Here's the drawing with two shaded views (mm, measured from the low corner). I have some questions. Coordinates: 2 decimals unless noted, no trailing zeros. Loops run counter-clockwise (first coordinate to the right, second up) from the corner with the lowest first, then second, coordinate; pieces in that order, holes last. Notation, with made-up numbers: M 42.5,43.5 L 80.5,43.5 A20 cw 80.5,50.5 Z; hole C 88.25,-2 d6. An arc over 180 degrees is marked long. Return JSON: item names as keys, results as strings. Group by question number.
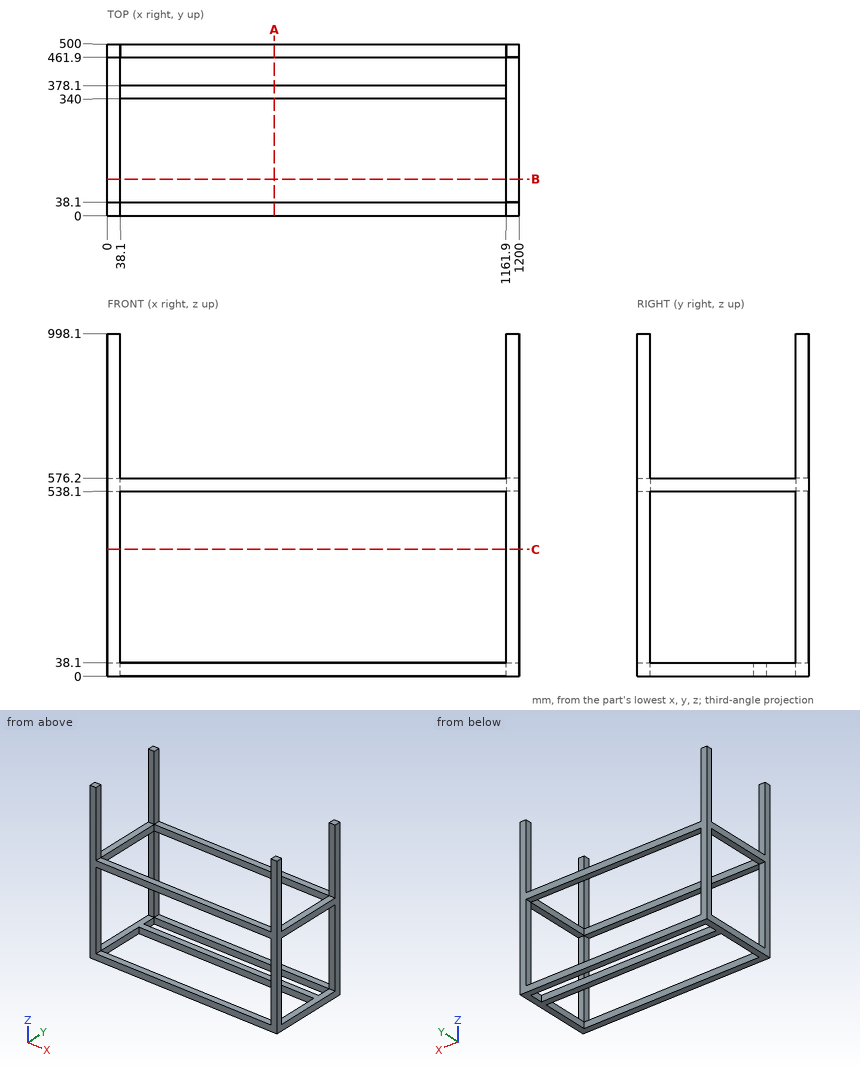
1) For pin 1 (11.5 mm diameter, centred on y = 26, z = 817, fed in from -X), with a flat end and sliding along its axis, tell me the tip position at first contact or that it passes through.
2) Suppose I cut it at C-C, the plane z = 369. List the corners of the cut face in (x, y) for me.
3) Suppose I cut it at B-B, the plane y = 106. List the corners of the cut face in (x, z) for me, then the cut area to 3 significant figures.
4) If I drill on line 1 (X direction, y = 402, z = 544); line 2 (Y direction, x = 425, z = 553.5), over which ranges is the centre line in solid material (lowest first)? Write a range as from..to.
5) Suppose I cut it at A-A, the plane x = 486.5. List the corners of the cut face in (y, z) for me, then the cut area to 3 significant figures.
Returned:
{
 "1": {"pin 1": "stops at x = 0"},
 "2": {"outline": "M 0,0 L 38.1,0 L 38.1,38.1 L 0,38.1 Z; M 0,461.9 L 38.1,461.9 L 38.1,500 L 0,500 Z; M 1161.9,0 L 1200,0 L 1200,38.1 L 1161.9,38.1 Z; M 1161.9,461.9 L 1200,461.9 L 1200,500 L 1161.9,500 Z"},
 "3": {"outline": "M 0,0 L 38.1,0 L 38.1,38.1 L 0,38.1 Z; M 0,538.1 L 38.1,538.1 L 38.1,576.2 L 0,576.2 Z; M 1161.9,0 L 1200,0 L 1200,38.1 L 1161.9,38.1 Z; M 1161.9,538.1 L 1200,538.1 L 1200,576.2 L 1161.9,576.2 Z", "area": "5,810 mm²"},
 "4": {"line 1": "x = 0..38.1, 1161.9..1200", "line 2": "y = 0..38.1, 461.9..500"},
 "5": {"outline": "M 0,0 L 38.1,0 L 38.1,38.1 L 0,38.1 Z; M 0,538.1 L 38.1,538.1 L 38.1,576.2 L 0,576.2 Z; M 340,0 L 378.1,0 L 378.1,38.1 L 340,38.1 Z; M 461.9,0 L 500,0 L 500,38.1 L 461.9,38.1 Z; M 461.9,538.1 L 500,538.1 L 500,576.2 L 461.9,576.2 Z", "area": "7,260 mm²"}
}
